Work out the finished part from the listing and answer in its coordinate system (mm). A direction names the side the tool comes from. Round coordinates to 2 decimals unless told otherwise and drop trailing zeros. Write each loop counter-clockwise with the first axis right and the second up, starting at its lowest first coordinate (ties: lowest second). Pieces come first, ordered by that corner, then holes. Notation, with made-up numbers: M 84.25,21 L 113.25,21 A33 ccw 113.25,59 Z; hole C -35,-7 d9. An arc over 180 degrees is marked long. One line per item, written item: value. Start each with the question number.
Q1. Find section B-B (z = -10). Write down the section's boundary in (x, y).
Q2. The mould has two halves that part along X. Classify faces 1 (the flat face through (0, 8, 2)), 2 (the cylindrical face through (2.604, -2.781, -6.261)), 3 (the flat face through (3, -3, 0)): released by +X, released by -X, zero draft, split by the parting line, or undercut.
Q3. Given pin 1 Ø3 at (y, z) = (-9, -3.5) entering from +X; pin 2 Ø4 at (x, y) = (6, 3) entering from +Z; pin 3 Ø1.1 at (y, z) = (-2.5, 2) entering from -X, each flat-ended and moving along its own axis, determine where each tip first touches the part or whether it passes through.
Q4. Find section C-C (y = 8.25). Write down the section's boundary in (x, z).
Q5. A tool of negligible diameter and unlimited length cuts with its end or side. For faces 4 (the flat face through (-10, 10, 0)), 5 (the flat face through (-6, 0, 2)), 6 (the cylindrical face through (3.81, 0.08, 1.88)), 7 (the flat face through (0, -2, 2)), from which of +Z, -Z, +X, -X, +Y, -Y can it reach the whole face along a straight path? Write none if from no direction.
Q6. Consider probe 1 along Y at (x, z) = (0, -3.5); probe 2 along Z at (x, y) = (5.25, 2); probe 3 along Y at (x, z) = (-2.5, -9.25). Determine where each line is inside the solid, lowest interval first.
Autodesk Inventor part; units mm, degrees
ref_plane "YZ Plane" through (0, 0, 0) normal (1, 0, 0) x (0, 1, 0)
ref_plane "XZ Plane" through (0, 0, 0) normal (0, 1, 0) x (-1, 0, 0)
ref_plane "XY Plane" through (0, 0, 0) normal (0, 0, 1) x (1, 0, 0)
sketch "Sketch1" plane through (0, 0, 0) normal (0, 0, 1) x (1, 0, 0)
  circle A0 centre (0, 0) radius 12.7
  circle A1 centre (0, 0) radius 3.81
  line L0 (0, 12.7) -> (0, 0)
  line L1 (0, 0) -> (12.7, 0)
  line L2 (0, -12.7) -> (0, 0)
  line L3 (-12.7, 0) -> (0, 0)
  line L4 (0, 3.81) -> (0, 0)
  line L5 (3.81, 0) -> (0, 0)
  line L6 (0, -3.81) -> (0, 0)
  line L7 (-3.81, 0) -> (0, 0)
  dimension "d0" = 25.4
  dimension "d1" = 7.62
extrude "Extrusion1" add sketch "Sketch1" against normal blind 12.7 contours L1 A1 L0 A0 | A0 L2 A1 L1 | L0 A1 L3 A0 | A0 L3 A1 L2
extrude "Extrusion2" cut sketch "Sketch1" against normal blind 12.7 contours L0 A1 L3 A0 | L0 L3 A1
sketch "Sketch2" plane through (0, 3.81, 0) normal (-1, 0, 0) x (0, 0, 1)
  line L0 (-12.7, 8.89) -> (-12.7, -16.51)
  line L1 (0, 0) -> (-12.7, 0)
  line L2 (-12.7, 8.89) -> (-12.7, 0)
  line L3 (-12.7, 0) -> (0, 0)
  line L4 (0, 8.89) -> (0, -16.51)
  line L5 (0, 0) -> (0, 8.89)
  line L6 (-12.7, 8.89) -> (0, 8.89)
  line L7 (0, 8.89) -> (-12.7, 8.89)
  point P0 (0, -3.81)
  point P1 (-12.7, -3.81)
extrude "Extrusion3" add sketch "Sketch2" along normal blind 12.7
extrude "Extrusion4" add sketch "Sketch1" along normal blind 3.81 contours A1 L2 L1 | L0 L3 A1
extrude "Extrusion5" add sketch "Sketch1" along normal blind 3.81 contours L1 L0 A1
extrude "Extrusion6" add sketch "Sketch1" along normal blind 3.81 contours L0 A1 L3 A0
properties part number "dope"
The answers:
1. outline: M -12.7,0 A12.7 ccw long 0,12.7 L -12.7,12.7 L -12.7,3.81 L 0,3.81 A3.81 cw long -3.81,0 Z
2. face 1: released by +X
2. face 2: undercut
2. face 3: zero draft
3. pin 1: x = 10.25
3. pin 2: z = 0
3. pin 3: x = 0
4. outline: M -12.7,-12.7 L 9.66,-12.7 L 9.66,0 L 0,0 L 0,3.81 L -9.66,3.81 L -9.66,0 L -12.7,0 Z
5. face 4: +Z, -X, +Y
5. face 5: +Z, -X, -Y
5. face 6: +Z, +X
5. face 7: +Z, -Z, -X, -Y
6. probe 1: -12.7 to -3.81, 3.81 to 12.7
6. probe 2: -12.7 to 0
6. probe 3: -12.45 to -2.88, 3.81 to 12.7
